The drawing under review shows one solid part. Ordinate dimensions are in mm from its lowest x, y, z. A direction names the side the tool comes from. Round coordinates to 2 decimals unless told otherwise and drop trailing zeros. Write each loop counter-clockwise with the first axis right and the second up, starting at its lowest first coordinate (ties: lowest second). Pieces come first, ordered by that corner, then holes.
Item 1: Add section C-C (y = 13.75). State how many separate pieces and enclosed holes the cut face has, plus the area to 3 significant figures.
Item 2: Machinability: for the marked faces 1 and 2, which of the approach directions +Z, -Z, +X, -X, +Y, -Y give a long, thin tool a straight path to every point of the face, cutting with its end or side? Answer none if there is none.
Item 3: Add section D-D (z = 7). Give the boundary of the cut face in (x, y).
Item 4: Add section B-B (z = 15.25). Give the boundary of the cut face in (x, y).
Item 5: Draft analysis for pull direction Y (two halves, no side actions). For the marked faces 3, 4, 5 and 6, state which applies: +Y half, -Y half, draft (parallel to the pull), parting line (faces both ways), or undercut.
Item 6: To check wall thickness, follow L1, parallel to Y at x = 7, z = 8.5; L2, parallel to X at y = 12.75, z = 9.75; L3, parallel to X at y = 18, z = 5.5 (1 decimal). State the ranges of each line that lie inside material, in increasing order.
Item 7: Add section A-A (x = 7). Give the boundary of the cut face in (y, z), plus the area to 3 significant figures.
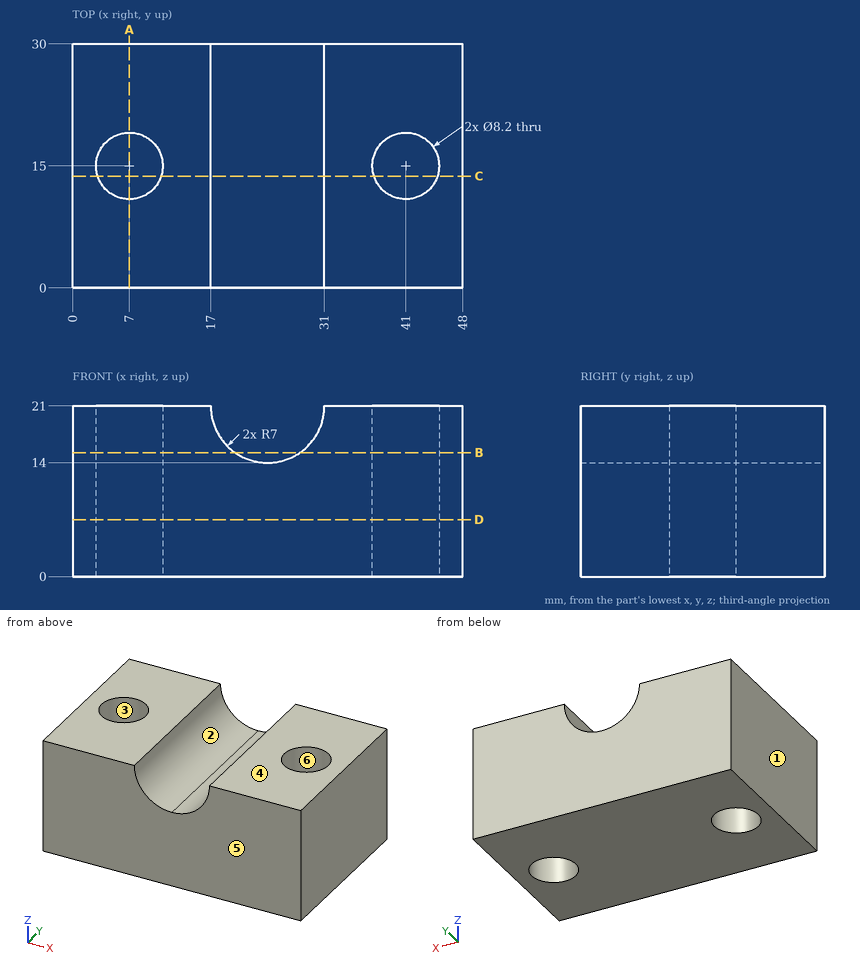
Numbers:
1. separate pieces: 3
1. enclosed holes: 0
1. area: 603 mm2
2. face 1: +Z, -Z, -X, +Y, -Y
2. face 2: +Z, +Y, -Y
3. outline: (0, 0) - (48, 0) - (48, 30) - (0, 30) - close; hole circle Ø8.2 at (7, 15); hole circle Ø8.2 at (41, 15)
4. outline: (0, 0) - (20.01, 0) - (20.01, 30) - (0, 30) - close; (27.99, 0) - (48, 0) - (48, 30) - (27.99, 30) - close; hole circle Ø8.2 at (7, 15); hole circle Ø8.2 at (41, 15)
5. face 3: undercut
5. face 4: draft
5. face 5: -Y half
5. face 6: undercut
6. L1: y = 0 to 10.9, 19.1 to 30
6. L2: x = 0 to 3.57, 10.43 to 37.57, 44.43 to 48
6. L3: x = 0 to 4.2, 9.8 to 38.2, 43.8 to 48
7. outline: (0, 0) - (10.9, 0) - (10.9, 21) - (0, 21) - close; (19.1, 0) - (30, 0) - (30, 21) - (19.1, 21) - close
7. area: 458 mm2
